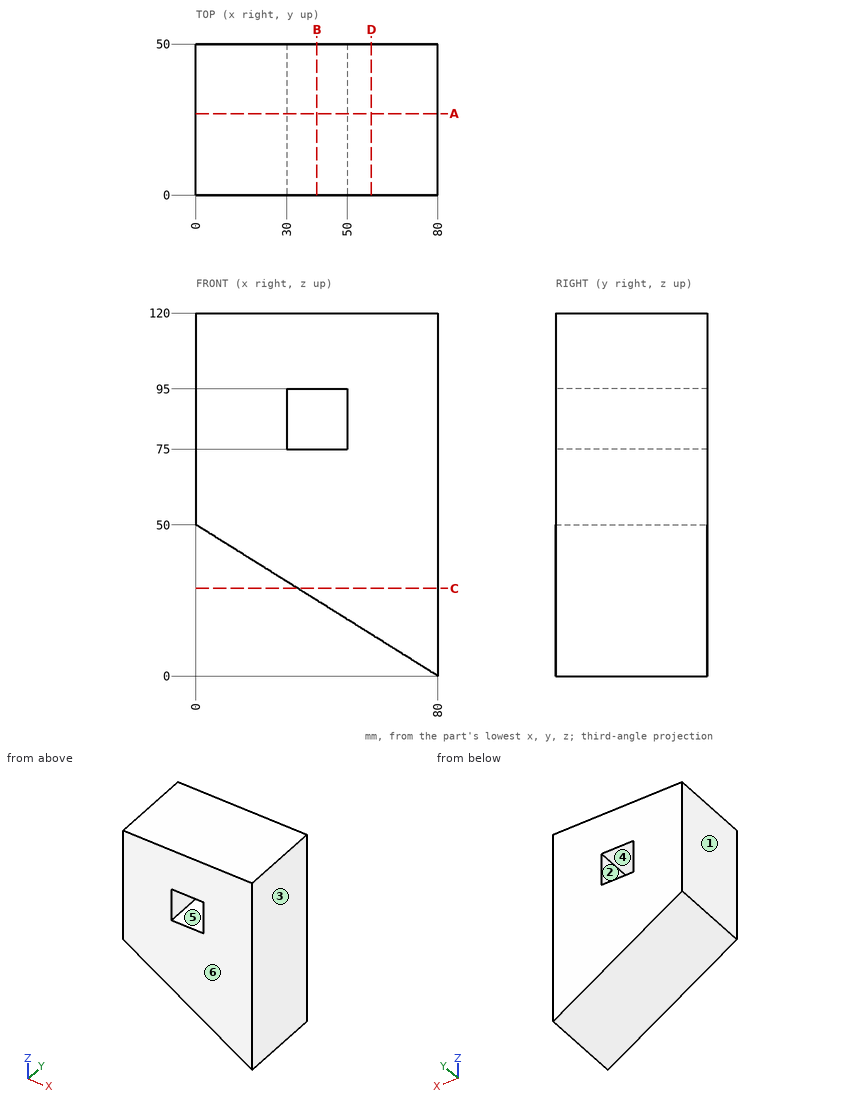
Drawing for the job (mm, zero at the part's lowest x, y, z). A direction names the side the tool comes from. Coordinates: 2 decimals unless noted, no trailing zeros. Order: outer loops, then holes, each group sorted by start corner. A loop starts at its lowest first (then second) coordinate and runs counter-clockwise, first axis right, second up.
Item 1: Two-plate mould, pull along X, no slides. Class the marked faces 1, 2, 3 and 4: +X half, -X half, draft (parallel to the pull), parting line (faces both ways), or undercut.
Check sheet entries:
face 1: -X half
face 2: undercut
face 3: +X half
face 4: undercut
Item 2: Band-saw the part on C-C on z = 29. List the corners of the cut face in (x, y), plus the area to 3 significant figures.
Check sheet entries:
outline: (33.6, 0) - (80, 0) - (80, 50) - (33.6, 50) - close
area: 2,320 mm2
Item 3: Band-saw the part on A-A on y = 27. List the corners of the cut face in (x, z).
Check sheet entries:
outline: (0, 50) - (80, 0) - (80, 120) - (0, 120) - close; hole (30, 75) - (50, 75) - (50, 95) - (30, 95) - close
Item 4: Band-saw the part on D-D on x = 58. List the corners of the cut face in (y, z).
Check sheet entries:
outline: (0, 13.75) - (50, 13.75) - (50, 120) - (0, 120) - close
Item 5: Pin check, flat tips, straight feed: pin 1 Ø6 at (x, y) = (33.5, 9) entering from -Z; pin 2 Ø1 at (x, y) = (54.5, 25) entering from -Z (3 decimals); pin 3 Ø10 at (x, y) = (43.5, 15) entering from -Z. Stop position of each tip, or through.
Check sheet entries:
pin 1: stops at z = 27.19
pin 2: stops at z = 15.625
pin 3: stops at z = 19.69
Item 6: 3-axis set-ups, long thin cutter, end or side, ignore diameter. For the marked faces 5 and 6: which of +Z, -Z, +X, -X, +Y, -Y reach the whole face in a straight line?
Check sheet entries:
face 5: +Y, -Y
face 6: +Z, -Z, +X, -X, -Y
Item 7: Band-saw the part on B-B on x = 40. List the corners of the cut face in (y, z), plus the area to 3 significant figures.
Check sheet entries:
outline: (0, 25) - (50, 25) - (50, 75) - (0, 75) - close; (0, 95) - (50, 95) - (50, 120) - (0, 120) - close
area: 3,750 mm2
Item 8: Drill centre lines: L1, parallel to X at y = 17, z = 76; L2, parallel to Z at x = 49, y = 42 (3 decimals); L3, parallel to X at y = 30, z = 26.5. Where is each one in solid material? Low to high.
Check sheet entries:
L1: x = 0 to 30, 50 to 80
L2: z = 19.375 to 75, 95 to 120
L3: x = 37.6 to 80
